from build123d import *

# Parameters (mm, degrees)
EXTRUDE_START   = 0.1
SKETCH_2_W      = 6
SKETCH_2_H      = 6
EXTRUDE_1_DEPTH = 3
CHAMFER_1_SIZE  = 1.18


with BuildPart() as part:
    # Эскиз1 → Повернуть1 (revolve)
    with BuildSketch(Plane.XY, mode=Mode.PRIVATE) as revolve_1_sk:
        with BuildLine():
            Line((25, 0), (25, 2.95))
            Line((25, 2.95), (7, 2.95))
            Line((7, 2.95), (7, 3))
            Line((7, 3), (0, 3))
            Line((0, 3), (0, 7))
            Line((0, 7), (-1.124355653, 7))
            ThreePointArc((-1.124355653, 7), (-2.522961568, 3.623466631), (-3, 0))
            Line((-3, 0), (25, 0))
        make_face()
    revolve(revolve_1_sk.sketch.rotate(Axis((-121.430503085, 0, 0), (1, 0, 0)), 90), axis=Axis((-121.430503085, 0, 0), (1, 0, 0)))

    # Эскиз2 → Бобышка-Вытянуть1 (add)
    with BuildSketch(Plane(origin=(0, 0, 0), x_dir=(0, 0, -1), z_dir=(1, 0, 0)).offset(EXTRUDE_START)):
        Rectangle(SKETCH_2_W, SKETCH_2_H)
    extrude(amount=EXTRUDE_1_DEPTH)

    # Фаска1
    chamfer_1_edges = [part.edges().sort_by_distance(p)[0] for p in [
        (25, 0, -2.95),
    ]]
    chamfer(chamfer_1_edges, length=CHAMFER_1_SIZE)


solid = part.part
Check sheet for the modelled part. Datum: model origin and axes. Units: mm. A direction names the side the tool comes from. Coordinates: 2 decimals unless noted, no trailing zeros. Loops run counter-clockwise (first coordinate to the right, second up) from the corner with the lowest first, then second, coordinate; pieces in that order, holes last. Notation, with made-up numbers: (4.25, 47.5) -> (15.25, 47.5) arc R11 ccw to (15.25, 57.5) -> close; hole circle Ø8 at (65, 72). An arc over 180 degrees is marked (long way). Answer in a Markdown table with one row per item.
1. Material ranges on line 1 along Y through (x, z) = (20.5, 0); line 2 along Z through (x, y) = (0.75, 2); line 3 along X through (y, z) = (-5.5, 3), recorded low to high. Write a range as [from, to].
Check values:
| item | result |
|---|---|
| line 1 | y = [-2.95, 2.95] |
| line 2 | z = [-3, 3] |
| line 3 | x = [-1.52, 0] |
2. Sectioned sample at B-B, the plane y = -3.5. Record the boundary of the cut face in (x, z), then the cut area to 3 significant figures.
Check values:
| item | result |
|---|---|
| outline | (-1.12, -6.06) -> (0, -6.06) -> (0, 6.06) -> (-1.12, 6.06) arc R13.56 ccw to start |
| area | 25.3 mm2 |
3. Access from +Z, -Z, +X, -X, +Y, -Y to the whole of each face (thin tool, end or side, straight path). Record for faces 1 (the face through (2, -3, 0)), 2 (the face through (3.1, -2.3, 2.4)), 3 (the face through (2, 3, 0)), 4 (the face through (2, 0, -3)).
Check values:
| item | result |
|---|---|
| face 1 | +Z, -Z, +X, -Y |
| face 2 | +Z, +X, -Y |
| face 3 | +Z, -Z, +X, +Y |
| face 4 | -Z, +X, +Y, -Y |
4. Sectioned sample at A-A, the plane x = 11. Record the boundary of the cut face in (y, z).
Check values:
| item | result |
|---|---|
| outline | circle Ø5.9 at (0, 0) |
5. Go/stop test with flat-tipped pins: pin 1 (1 mm diameter, centred on x = 7, z = 4, fed in from +Y); pin 2 (2.5 mm diameter, centred on x = 1, y = -1, fed in from +Z); pin 3 (2.5 mm diameter, centred on y = 2, z = 1.5, fed in from -X); pin 4 (4 mm diameter, centred on x = 20, y = 2.5, fed in from -Z). Record where each tip stops, or that it passes through.
Check values:
| item | result |
|---|---|
| pin 1 | passes through |
| pin 2 | stops at z = 7 |
| pin 3 | stops at x = -2.94 |
| pin 4 | stops at z = -2.91 |
6. Sectioned sample at C-C, the plane z = -5.25. Record the boundary of the cut face in (x, y), then the cut area to 3 significant figures.
Check values:
| item | result |
|---|---|
| outline | (-1.12, -4.63) -> (0, -4.63) -> (0, 4.63) -> (-1.12, 4.63) arc R12.98 ccw to start |
| area | 15.7 mm2 |
